Verification items for the finished model (mm, model axes). Face numbers are marked on the shaded views. A direction names the side the tool comes from. Give positions to 0.01 mm unless a question says otherwise; leave off trailing zeros. Write each loop counter-clockwise with the first axis right and the second up, starting at its lowest first coordinate (ties: lowest second). Pieces come first, ordered by that corner, then holes. Notation, with made-up numbers: M -39,-18 L 3,-18 A9 ccw 3,-10 Z; hole C -36.5,55 d4. An arc over 180 degrees is marked long. Answer as a JSON object with one key per item and string values.
```python
from build123d import *

# Parameters (mm, degrees)
F0_R     = 12.5
F0_R_2   = 3
F1_DEPTH = 4
F2_DEPTH = 2
F5_R     = 5


with BuildPart() as f1:
    # F0 (on Top) → F1 (new body)
    with BuildSketch(Plane.XY):
        Circle(F0_R)
        Circle(F0_R_2, mode=Mode.SUBTRACT)
        Circle(F0_R_2)
    extrude(amount=F1_DEPTH)

    # F0 (on Top) → F2 (cut)
    with BuildSketch(Plane.XY):
        Circle(F0_R_2)
    extrude(amount=F2_DEPTH, mode=Mode.SUBTRACT)

    # F3 (on Front) → F4 (revolve, cut)
    with BuildSketch(Plane.XZ):
        with BuildLine():
            ThreePointArc((0, 153.5), (-75, 78.5), (0, 3.5))
            Line((0, 3.5), (0, 4))
            Line((0, 4), (0, 153.5))
        make_face()
    revolve(axis=Axis((0, 0, 82.6326791644), (0, 0, 1)), mode=Mode.SUBTRACT)

    # F5
    f5_edges = [f1.edges().sort_by_distance(p)[0] for p in [
        (8.645808, 0, 4),
    ]]
    fillet(f5_edges, radius=F5_R)


solid = f1.part
```
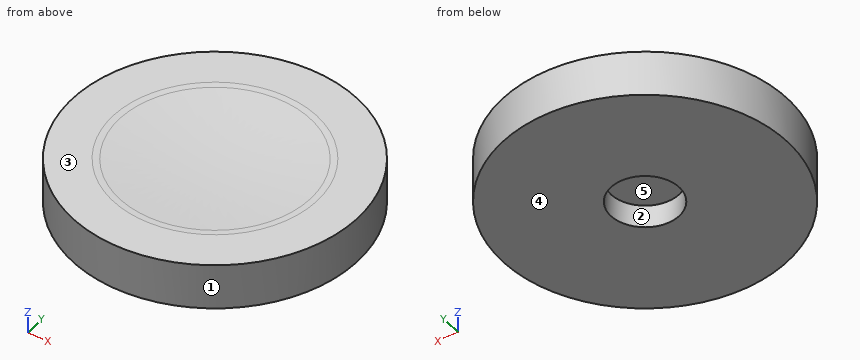
1) Access from +Z, -Z, +X, -X, +Y, -Y to the whole of each face (thin tool, end or side, straight path). Record for the marked faces 4 and 5.
Completed:
{"face 4": "-Z, +X, -X, +Y, -Y", "face 5": "-Z"}
2) Go/stop test with flat-tipped pins: pin 1 (6 mm diameter, centred on x = -6.5, y = -6.5, fed in from -Z); pin 2 (3.5 mm diameter, centred on x = 0, y = 0, fed in from +Z); pin 3 (1.8 mm diameter, centred on x = -0.5, y = 1, fed in from -Z). Record where each tip stops, or that it passes through.
Completed:
{"pin 1": "stops at z = 0", "pin 2": "stops at z = 3.52", "pin 3": "stops at z = 2"}
3) Section check B-B on z = 0.3. Record the boundary of the cut face in (x, y).
Completed:
{"outline": "C 0,0 d25; hole C 0,0 d6"}
4) Section check A-A on y = -10. Record the boundary of the cut face in (x, z).
Completed:
{"outline": "M -7.5,0 L 7.5,0 L 7.5,4 L -7.5,4 Z"}
5) Release check for a two-part mould opening along Y. For the marked faces 1, 2 and 3 record: pulls with the +Y half, pulls with the -Y half, needs draft (parallel to the pull), parting line crosses it, or undercut.
Completed:
{"face 1": "parting line crosses it", "face 2": "undercut", "face 3": "needs draft"}
6) Thickness scan on L1, parallel to Y at x = 0, z = 0.5; L2, parallel to Y at x = 5.5, z = 0.6; L3, parallel to X at y = 0.5, z = 0.35. Record the ranges inside material, lowest first.
Completed:
{"L1": "y = -12.5 to -3, 3 to 12.5", "L2": "y = -11.22 to 11.22", "L3": "x = -12.49 to -2.96, 2.96 to 12.49"}
7) Section check C-C on z = 3.2. Record the boundary of the cut face in (x, y).
Completed:
{"outline": "C 0,0 d25"}
